```python
from build123d import *

# Parameters (mm, degrees)
SKETCH1_R                                    = 10
BOSS_EXTRUDE1_DEPTH                          = 1.5
SKETCH2_R                                    = 10
SKETCH2_R_2                                  = 7.5
BOSS_EXTRUDE2_DEPTH                          = 1
CSK_FOR_M3_COUNTERSUNK_FLAT_HEAD_SCR_2_COUNT = 2
CSK_FOR_M3_COUNTERSUNK_FLAT_HEAD_SCR_2_PITCH = 8.485281374
CSK_FOR_M3_COUNTERSUNK_FLAT_HEAD_SCR_3_COUNT = 2
CSK_FOR_M3_COUNTERSUNK_FLAT_HEAD_SCR_3_PITCH = 12
CSK_FOR_M3_COUNTERSUNK_FLAT_HEAD_SCR_4_COUNT = 2
CSK_FOR_M3_COUNTERSUNK_FLAT_HEAD_SCR_4_PITCH = 8.485281374
SKETCH5_R                                    = 3.15
CUT_EXTRUDE1_DEPTH                           = 21
SKETCH6_R                                    = 2.5
CUT_EXTRUDE2_DEPTH                           = 2
CUT_EXTRUDE2_DEPTH_BACK                      = 2.5


with BuildPart() as part:
    # Sketch1 → Boss-Extrude1 (new body)
    with BuildSketch(Plane(origin=(0, 0, 0), x_dir=(1, 0, 0), z_dir=(0, 1, 0))):
        Circle(SKETCH1_R)
    extrude(amount=BOSS_EXTRUDE1_DEPTH)

    # Sketch2 → Boss-Extrude2 (add)
    with BuildSketch(Plane(origin=(0, 1.5, 0), x_dir=(1, 0, 0), z_dir=(0, 1, 0))):
        Circle(SKETCH2_R)
        Circle(SKETCH2_R_2, mode=Mode.SUBTRACT)
    extrude(amount=BOSS_EXTRUDE2_DEPTH)

    # Sketch4 → CSK for M3 Countersunk Flat Head Screw1 (revolve, cut)
    with BuildSketch(Plane(origin=(-6, 1.5, 0), x_dir=(0, 0, 1), z_dir=(1, 0, 0))):
        Polygon((0, 0), (0, 1.5), (1.7, 1.5), (1.7, 1.45), (3.15, 0), align=None)
    csk_for_m3_countersunk_flat_head_screw1 = revolve(axis=Axis((-6, 7.85, 0), (0, -1, 0)), mode=Mode.SUBTRACT)

    # CSK for M3 Countersunk Flat Head Scr 2: CSK for M3 Countersunk Flat Head Screw1 ×2
    with Locations(*[Vector(0.707106781, 0, -0.707106781) * (i * CSK_FOR_M3_COUNTERSUNK_FLAT_HEAD_SCR_2_PITCH) for i in range(1, CSK_FOR_M3_COUNTERSUNK_FLAT_HEAD_SCR_2_COUNT)]):
        add(csk_for_m3_countersunk_flat_head_screw1, mode=Mode.SUBTRACT)

    # CSK for M3 Countersunk Flat Head Scr 3: CSK for M3 Countersunk Flat Head Screw1 ×2
    with Locations(*[(i * CSK_FOR_M3_COUNTERSUNK_FLAT_HEAD_SCR_3_PITCH, 0, 0) for i in range(1, CSK_FOR_M3_COUNTERSUNK_FLAT_HEAD_SCR_3_COUNT)]):
        add(csk_for_m3_countersunk_flat_head_screw1, mode=Mode.SUBTRACT)

    # CSK for M3 Countersunk Flat Head Scr 4: CSK for M3 Countersunk Flat Head Screw1 ×2
    with Locations(*[Vector(0.707106781, 0, 0.707106781) * (i * CSK_FOR_M3_COUNTERSUNK_FLAT_HEAD_SCR_4_PITCH) for i in range(1, CSK_FOR_M3_COUNTERSUNK_FLAT_HEAD_SCR_4_COUNT)]):
        add(csk_for_m3_countersunk_flat_head_screw1, mode=Mode.SUBTRACT)

    # Sketch5 → Cut-Extrude1 (cut)
    with BuildSketch(Plane(origin=(0, 1.5, 0), x_dir=(1, 0, 0), z_dir=(0, 1, 0))):
        with Locations((6, 0)):
            Circle(SKETCH5_R)
        with Locations((0, -6)):
            Circle(SKETCH5_R)
        with Locations((-6, 0)):
            Circle(SKETCH5_R)
        with Locations((0, 6)):
            Circle(SKETCH5_R)
    extrude(amount=CUT_EXTRUDE1_DEPTH, mode=Mode.SUBTRACT)

    # Sketch6 → Cut-Extrude2 (cut, two sides)
    with BuildSketch(Plane(origin=(0, 1.5, 0), x_dir=(1, 0, 0), z_dir=(0, 1, 0))) as cut_extrude2_sk:
        Circle(SKETCH6_R)
    extrude(amount=CUT_EXTRUDE2_DEPTH, mode=Mode.SUBTRACT)
    extrude(cut_extrude2_sk.sketch, amount=-CUT_EXTRUDE2_DEPTH_BACK, mode=Mode.SUBTRACT)


solid = part.part
```
Can you work these out from the model? Positions are in its coordinate system, mm. A direction names the side the tool comes from. Give positions to 0.01 mm unless a question says otherwise; leave off trailing zeros. Loops run counter-clockwise (first coordinate to the right, second up) from the corner with the lowest first, then second, coordinate; pieces in that order, holes last. Notation, with made-up numbers: M 16,-9 L 58,-9 A16 cw 58,18 Z; hole C 83,75.5 d11. An arc over 180 degrees is marked long. Answer in a Markdown table with one row per item.
1. Suppose I cut it at B-B on z = 0. Write out the boundary of the cut face in (x, y), plus the area to 4 significant figures.
Taken from the geometry:
| item | result |
|---|---|
| outline | M -10,0 L -7.7,0 L -7.7,0.05 L -9.15,1.5 L -9.15,2.5 L -10,2.5 Z; M -4.3,0 L -2.5,0 L -2.5,1.5 L -2.85,1.5 L -4.3,0.05 Z; M 2.5,0 L 4.3,0 L 4.3,0.05 L 2.85,1.5 L 2.5,1.5 Z; M 7.7,0 L 10,0 L 10,2.5 L 9.15,2.5 L 9.15,1.5 L 7.7,0.05 Z |
| area | 9.795 mm² |
2. If I drill on line 1 along X through (y, z) = (0.3, 0.25); line 2 along X through (y, z) = (0.45, 0); line 3 along Z through (x, y) = (0, 0.4), over which ranges is the centre line in solid material (lowest first)?
Taken from the geometry:
| item | result |
|---|---|
| line 1 | x = -10 to -7.93, -4.07 to -2.49, 2.49 to 4.07, 7.93 to 10 |
| line 2 | x = -10 to -8.1, -3.9 to -2.5, 2.5 to 3.9, 8.1 to 10 |
| line 3 | z = -10 to -8.05, -3.95 to -2.5, 2.5 to 3.95, 8.05 to 10 |
3. Thinking about a two-plate mould opening in X: for faces 3 (the flat face through (-4, 2.5, 7)), 4 (the cylindrical face through (0.06, 1.99, -9.15)), 5 (the cylindrical face through (-2.17, 1.23, 9.76)), which applies, released by +X, released by -X, zero draft, split by the parting line, or undercut?
Taken from the geometry:
| item | result |
|---|---|
| face 3 | zero draft |
| face 4 | undercut |
| face 5 | split by the parting line |
4. Suppose I cut it at D-D on y = 2.1. Write out the boundary of the cut face in (x, z), plus the area to 3 significant figures.
Taken from the geometry:
| item | result |
|---|---|
| outline | C 0,0 d20; hole M -6.86,-3.03 A7.5 ccw -3.03,-6.86 A3.15 ccw 3.03,-6.86 A7.5 ccw 6.86,-3.03 A3.15 ccw 6.86,3.03 A7.5 ccw 3.03,6.86 A3.15 ccw -3.03,6.86 A7.5 ccw -6.86,3.03 A3.15 ccw Z |
| area | 107 mm² |
5. Suppose I cut it at C-C on z = 6. Write out the boundary of the cut face in (x, y), plus the area to 3 significant figures.
Taken from the geometry:
| item | result |
|---|---|
| outline | M -8,0 L -1.7,0 L -1.7,0.05 L -3.15,1.5 L -4.5,1.5 L -4.5,2.5 L -8,2.5 Z; M 1.7,0 L 8,0 L 8,2.5 L 4.5,2.5 L 4.5,1.5 L 3.15,1.5 L 1.7,0.05 Z |
| area | 23.8 mm² |
6. Suppose I cut it at A-A on x = -6. Write out the boundary of the cut face in (y, z), plus the area to 3 significant figures.
Taken from the geometry:
| item | result |
|---|---|
| outline | M 0,-8 L 2.5,-8 L 2.5,-4.5 L 1.5,-4.5 L 1.5,-3.15 L 0.05,-1.7 L 0,-1.7 Z; M 0,1.7 L 0.05,1.7 L 1.5,3.15 L 1.5,4.5 L 2.5,4.5 L 2.5,8 L 0,8 Z |
| area | 23.8 mm² |
7. Which directions (+Z, -Z, +X, -X, +Y, -Y) give clear straight access to the entire face, cutting with the end or side of a thin tool? Please do faces 1 (the cylindrical face through (5.331, 1.993, -5.276)), 2 (the flat face through (2, 0, 2)).
Taken from the geometry:
| item | result |
|---|---|
| face 1 | +Y |
| face 2 | +Z, -Z, +X, -X, -Y |
8. For pin 1 Ø4.5 at (x, z) = (6, 0) entering from +Y; pin 2 Ø1.5 at (x, y) = (-5, 1.5) entering from +Z; pin 3 Ø6.5 at (x, z) = (0, 0) entering from +Y, each with a flat end and sliding along its axis, tell me the tip position at first contact or that it passes through.
Taken from the geometry:
| item | result |
|---|---|
| pin 1 | stops at y = 0.6 |
| pin 2 | stops at z = 9.05 |
| pin 3 | stops at y = 1.5 |
